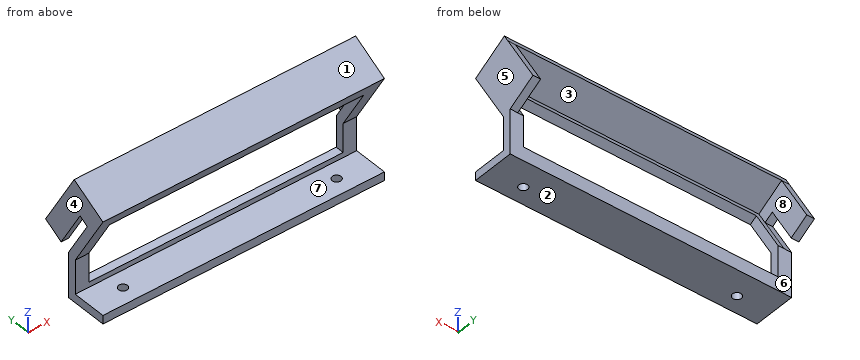
```python
from build123d import *

# Parameters (mm, degrees)
BOSS_EXTRUDE1_DEPTH = 83
SKETCH2_W           = 4.5
SKETCH2_H           = 36.339745962
BOSS_EXTRUDE2_DEPTH = 19
SKETCH3_W           = 150
SKETCH3_H           = 18.339745962
CUT_EXTRUDE1_DEPTH  = 6
SKETCH4_W           = 150
SKETCH4_H           = 31.34
CUT_EXTRUDE2_DEPTH  = 5
CUT_EXTRUDE3_DEPTH  = 5
SKETCH6_R           = 2.6
CUT_EXTRUDE4_DEPTH  = 5


with BuildPart() as part:
    # Sketch1 → Boss-Extrude1 (new, symmetric)
    with BuildSketch(Plane(origin=(0, 0, 0), x_dir=(0, 0, -1), z_dir=(1, 0, 0))):
        Polygon((0, 0), (0, 20), (-20, 20), (-54.641016151, 0), (-66.641016151, 20.784609691), (-62.310889132, 23.284609691), (-52.810889132, 6.830127019), (-21.339745962, 25), (5, 25), (5, 0), align=None)
    extrude(amount=BOSS_EXTRUDE1_DEPTH, both=True)

    # Sketch2 → Boss-Extrude2 (add)
    with BuildSketch(Plane(origin=(0, 27.990381057, 16.160254038), x_dir=(1, 0, 0), z_dir=(0, 0.866025403784436, 0.5000000000000044))):
        with Locations((-80.75, -24.150635095)):
            Rectangle(SKETCH2_W, SKETCH2_H)
        with Locations((80.75, -24.150635095)):
            Rectangle(SKETCH2_W, SKETCH2_H)
    extrude(amount=BOSS_EXTRUDE2_DEPTH)

    # Sketch3 → Cut-Extrude1 (cut)
    with BuildSketch(Plane(origin=(0, 25, 0), x_dir=(1, 0, 0), z_dir=(0, 1, 0))):
        with Locations((0, -12.169872981)):
            Rectangle(SKETCH3_W, SKETCH3_H)
    extrude(amount=-CUT_EXTRUDE1_DEPTH, mode=Mode.SUBTRACT)

    # Sketch4 → Cut-Extrude2 (cut)
    with BuildSketch(Plane(origin=(0, 27.990381057, 16.160254038), x_dir=(1, 0, 0), z_dir=(0, 0.8660254037844362, 0.5000000000000046))):
        with Locations((0, -21.650762114)):
            Rectangle(SKETCH4_W, SKETCH4_H)
    extrude(amount=-CUT_EXTRUDE2_DEPTH, mode=Mode.SUBTRACT)

    # Sketch5 → Cut-Extrude3 (cut)
    with BuildSketch(Plane.ZY.offset(83)):
        Polygon((21.339745962, 25), (45.016880502, 11.33), (48.016880502, 16.526152423), (24.339745962, 30.196152423), align=None)
    extrude(amount=-CUT_EXTRUDE3_DEPTH, mode=Mode.SUBTRACT)

    # Sketch6 → Cut-Extrude4 (cut)
    with BuildSketch(Plane(origin=(0, 0, -5), x_dir=(-1, 0, 0), z_dir=(0, 0, -1))):
        with Locations((-63, 10)):
            Circle(SKETCH6_R)
        with Locations((63, 10)):
            Circle(SKETCH6_R)
    extrude(amount=-CUT_EXTRUDE4_DEPTH, mode=Mode.SUBTRACT)


solid = part.part
```
CAD build for the part. Positions are in the model's coordinates, mm. Face numbers are marked on the shaded views. A direction names the side the tool comes from. Round coordinates to 2 decimals unless told otherwise and drop trailing zeros. Loops run counter-clockwise (first coordinate to the right, second up) from the corner with the lowest first, then second, coordinate; pieces in that order, holes last. Notation, with made-up numbers: (26, -22) - (60, -22) arc R24 ccw to (60, 12) - close; hole circle Ø9 at (-27.75, 33.25). An arc over 180 degrees is marked (long way). Return JSON: item names as keys, results as strings. Group by question number.
Q1. Drill centre lines: line 1 along Y through (x, z) = (63, -1.8); line 2 along X through (y, z) = (11.5, 44.5); line 3 along X through (y, z) = (21, 45). Where is each one in solid material? Low to high. Write a range as [from, to].
Q2. Band-saw the part on A-A on x = -63. Give the cut face in (y, z).
Q3. Band-saw the part on B-B on x = 20.5. Give the cut face in (y, z), plus the area to 3 significant figures.
Q4. Band-saw the part on C-C on y = 38. Give the cut face in (x, z).
Q5. Two-plate mould, pull along Z, no slides. Class the marked faces 1, 2 and 3: +Z half, -Z half, draft (parallel to the pull), parting line (faces both ways), or undercut.
Q6. Band-saw the part on D-D on z = 42. Give the cut face in (x, y).
Q7. Flat gauge pins, fed straight in: pin 1 Ø21 at (x, z) = (-31, 11) entering from +Y; pin 2 Ø16 at (x, y) = (25.5, 13.5) entering from +Z; pin 3 Ø6 at (x, y) = (63, 10) entering from +Z. Where does each tip first touch, or does it go through?
Q8. Tool access for the marked faces 4, 5, 6, 7 and 8: list every direction of +Z, -Z, +X, -X, +Y, -Y with a clear straight run to the whole face (end or side of a thin tool).
Solutions:
{
 "1": {"line 1": "y = [0, 7.4], [12.6, 25]", "line 2": "x = [-83, -75], [75, 83]", "line 3": "x = [-83, -78.5], [78.5, 83]"},
 "2": {"outline": "(0, -5) - (7.4, -5) - (7.4, 0) - (0, 0) - close; (0, 54.64) - (5, 45.98) - (9.33, 48.48) - (6.83, 52.81) - (23.28, 62.31) - (20.78, 66.64) - close; (12.6, -5) - (25, -5) - (25, 3) - (20, 3) - (20, 0) - (12.6, 0) - close"},
 "3": {"outline": "(0, -5) - (25, -5) - (25, 3) - (20, 3) - (20, 0) - (0, 0) - close; (0, 54.64) - (5, 45.98) - (9.33, 48.48) - (6.83, 52.81) - (23.28, 62.31) - (20.78, 66.64) - close", "area": "285 mm^2"},
 "4": {"outline": "(-83, 28.85) - (-78.5, 28.85) - (-78.5, 36.82) - (-83, 36.82) - close; (78.5, 28.85) - (83, 28.85) - (83, 36.82) - (78.5, 36.82) - close"},
 "5": {"face 1": "+Z half", "face 2": "-Z half", "face 3": "undercut"},
 "6": {"outline": "(-83, 7.3) - (-75, 7.3) - (-75, 13.07) - (-83, 13.07) - close; (-83, 20) - (-78.5, 20) - (-78.5, 35.01) - (-83, 35.01) - close; (75, 7.3) - (83, 7.3) - (83, 35.01) - (78.5, 35.01) - (78.5, 13.07) - (75, 13.07) - close"},
 "7": {"pin 1": "stops at y = 25", "pin 2": "stops at z = 66.64", "pin 3": "stops at z = 62.15"},
 "8": {"face 4": "+Z, -Z, -X, +Y, -Y", "face 5": "+Z, -Z, +X, +Y, -Y", "face 6": "-Z, +X, -X, +Y", "face 7": "+X, -X, -Y", "face 8": "+Y"}
}
